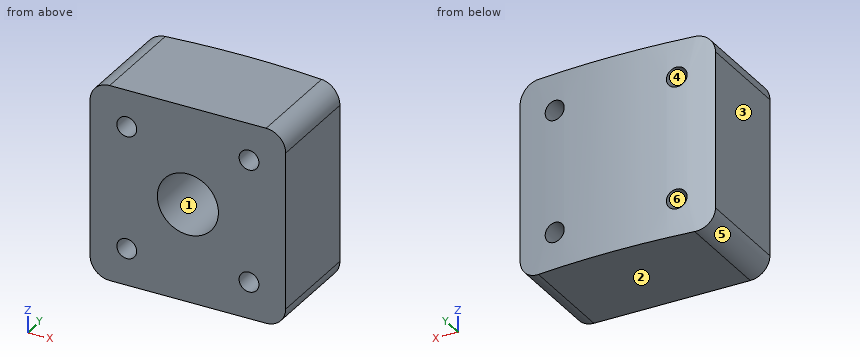
```python
from build123d import *

# Parameters (mm, degrees)
BOSS_EXTRUDE1_DEPTH             = 12.7
BOSS_EXTRUDE1_DEPTH_BACK        = 12.7
TAP_DRILL_FOR_3_8_16_TAP1_D     = 7.9375
TAP_DRILL_FOR_3_8_16_TAP1_DEPTH = 9.525
TAP_DRILL_FOR_3_8_16_TAP1_TIP   = 2.384665582
F_5_40_TAPPED_HOLE1_D           = 2.5781
FILLET1_R                       = 2.54


with BuildPart() as part:
    # Sketch1 → Boss-Extrude1 (new, two sides: drawn at the far end of the back side and taken through both)
    with BuildSketch(Plane.XY.offset(-BOSS_EXTRUDE1_DEPTH_BACK)):
        with BuildLine():
            Line((-12.701329683, 100.803292467), (-12.701329683, 88.103292467))
            Line((-12.701329683, 88.103292467), (12.698670317, 88.103292467))
            Line((12.698670317, 88.103292467), (12.698670317, 100.749441262))
            ThreePointArc((12.698670317, 100.749441262), (0.000359797, 101.573243718), (-12.701329683, 100.803292467))
        make_face()
    extrude(amount=BOSS_EXTRUDE1_DEPTH + BOSS_EXTRUDE1_DEPTH_BACK)

    # Tap Drill for 3/8-16 Tap1
    with Locations(Plane(origin=(0, 88.103292467, 0), x_dir=(-1, 0, 0), z_dir=(0, -1, 0))):
        with Locations((0, 0)):
            Hole(TAP_DRILL_FOR_3_8_16_TAP1_D / 2, depth=TAP_DRILL_FOR_3_8_16_TAP1_DEPTH)
            with Locations((0, 0, -(TAP_DRILL_FOR_3_8_16_TAP1_DEPTH + TAP_DRILL_FOR_3_8_16_TAP1_TIP / 2))):  # 118° drill point
                Cone(0, TAP_DRILL_FOR_3_8_16_TAP1_D / 2, TAP_DRILL_FOR_3_8_16_TAP1_TIP, mode=Mode.SUBTRACT)

    # #5-40 Tapped Hole1 (through all)
    with Locations(Plane(origin=(0, 88.103292467, 0), x_dir=(-1, 0, 0), z_dir=(0, -1, 0))):
        with Locations((-7.9375, -7.9375), (-7.9375, 7.9375), (7.9375, 7.9375), (7.9375, -7.9375)):
            Hole(F_5_40_TAPPED_HOLE1_D / 2)

    # Fillet1
    fillet1_edges = [part.edges().sort_by_distance(p)[0] for p in [
        (-12.701329683, 94.453292467, 12.7),
        (12.698670317, 94.426366864, -12.7),
        (12.698670317, 94.426366864, 12.7),
        (-12.701329683, 94.453292467, -12.7),
    ]]
    fillet(fillet1_edges, radius=FILLET1_R)


solid = part.part
```
Input: part model. Units: mm. Frame: model coordinates. Face numbers are marked on the shaded views. A direction names the side the tool comes from. Round coordinates to 2 decimals unless told otherwise and drop trailing zeros. Order: outer loops, then holes, each group sorted by start corner. A loop starts at its lowest first (then second) coordinate and runs counter-clockwise, first axis right, second up. Notation, with made-up numbers: (57.25, 29) - (71.25, 29) arc R28 ccw to (71.25, 59) - close; hole circle Ø4 at (63.5, 63). An arc over 180 degrees is marked (long way). One line per question, with ' | ' between items. Start each with the question number.
1) Cut plane A-A, the plane z = 8.5. Return the cut outline in (x, y), then the cut area to 3 significant figures.
2) Set-up query: the marked faces 1 and 2. Return all of +Z, -Z, +X, -X, +Y, -Y with unobstructed straight access to the full face (end or side cutting, diameter ignored); none if empty.
3) Pull-direction query (Z, two-part tool) for the marked faces 3, 4, 5 and 6; classes: +Z half, -Z half, draft (parallel to the pull), parting line (faces both ways), or undercut.
4) Cut plane B-B, the plane x = -8.5. Return the cut outline in (y, z), then the cut area to 3 significant figures.
5) Contact query for a flat-ended pin moving along its axis: P1, Ø4, axis at x = 7.94, z = 7.94, coming from the +Y side. Output: stop coordinate, or through.
6) Ray query, probe 1 along Z at (x, y) = (0, 95.75); probe 2 along X at (y, z) = (93.75, 7.5); probe 3 along Z at (x, y) = (8.25, 91.75). Return the intervals inside material, ascending.
7) Cut plane C-C, the plane y = 95.25. Return the cut outline in (x, z), then the cut area to 3 significant figures.
Worked out:
1) outline: (-12.7, 88.1) - (-9.1, 88.1) - (-9.1, 101.18) arc R101.6 ccw to (-12.7, 100.8) - close; (-6.78, 88.1) - (6.78, 88.1) - (6.78, 101.33) arc R101.6 ccw to (-6.78, 101.36) - close; (9.1, 88.1) - (12.7, 88.1) - (12.7, 100.75) arc R101.6 ccw to (9.1, 101.15) - close | area: 274 mm^2
2) face 1: -Y | face 2: -Z, +X, -X, +Y, -Y
3) face 3: draft | face 4: undercut | face 5: -Z half | face 6: undercut
4) outline: (88.1, -12.7) - (101.24, -12.7) - (101.24, -9.1) - (88.1, -9.1) - close; (88.1, -6.78) - (101.24, -6.78) - (101.24, 6.78) - (88.1, 6.78) - close; (88.1, 9.1) - (101.24, 9.1) - (101.24, 12.7) - (88.1, 12.7) - close | area: 273 mm^2
5) P1: stops at y = 101.39
6) probe 1: z = -12.7 to -3.97, 3.97 to 12.7 | probe 2: x = -12.7 to -9.15, -6.72 to 6.72, 9.15 to 12.7 | probe 3: z = -12.7 to -9.19, -6.69 to 6.69, 9.19 to 12.7
7) outline: (-12.7, -10.16) arc R2.54 ccw to (-10.16, -12.7) - (10.16, -12.7) arc R2.54 ccw to (12.7, -10.16) - (12.7, 10.16) arc R2.54 ccw to (10.16, 12.7) - (-10.16, 12.7) arc R2.54 ccw to (-12.7, 10.16) - close; hole circle Ø2.58 at (-7.94, -7.94); hole circle Ø2.58 at (-7.94, 7.94); hole circle Ø7.94 at (0, 0); hole circle Ø2.58 at (7.94, -7.94); hole circle Ø2.58 at (7.94, 7.94) | area: 569 mm^2
